Design review of the part built by this model. Coordinates are the model's own, in mm. A direction names the side the tool comes from. Coordinates: 2 decimals unless noted, no trailing zeros. Order: outer loops, then holes, each group sorted by start corner. A loop starts at its lowest first (then second) coordinate and runs counter-clockwise, first axis right, second up. Notation, with made-up numbers: (54, 60.25) - (100, 60.25) arc R19 ccw to (100, 85.25) - close; hole circle Ø8 at (-4, -30). An arc over 180 degrees is marked (long way). Write item = value, one per line. Start each with the question number.
```python
from build123d import *
from OCP.BRepFilletAPI import BRepFilletAPI_MakeChamfer

# Parameters (mm, degrees)
AUFSATZ_LINEAR_AUSTRAGEN1_DEPTH = 45
FASE1_SIZE                      = 35
FASE1_SIZE2                     = 50
FASE2_SIZE                      = 35
FASE2_SIZE2                     = 5
SCHNITT_LINEAR_AUSTRAGEN2_DEPTH = 140.810416962
SKIZZE4_W                       = 210
SKIZZE4_H                       = 7
AUFSATZ_LINEAR_AUSTRAGEN2_DEPTH = 10
VERRUNDUNG2_R                   = 3.5
VERRUNDUNG3_R                   = 3


with BuildPart() as part:
    # Skizze1 → Aufsatz-Linear austragen1 (new body)
    with BuildSketch(Plane(origin=(0, 0, 0), x_dir=(1, 0, 0), z_dir=(0, 1, 0))):
        Polygon((-105, -55), (-105, 0), (105, 0), (105, -55), (110, -55), (120.403291862, 4), (-120.403291862, 4), (-110, -55), align=None)
    extrude(amount=AUFSATZ_LINEAR_AUSTRAGEN1_DEPTH)

    # Fase1: one chamfer whose edges measure the first distance from different faces: ONE call of the kernel's chamfer builder (chamfer() names one face for all edges)
    fase1_edges_1 = [part.edges().sort_by_distance(p)[0] for p in [
        (107.5, 45, 55),
    ]]
    fase1_side_1 = [part.faces().sort_by_distance(p)[0] for p in [
        (107.5, 22.5, 55),
    ]]
    fase1_edges_2 = [part.edges().sort_by_distance(p)[0] for p in [
        (-107.5, 45, 55),
    ]]
    fase1_side_2 = [part.faces().sort_by_distance(p)[0] for p in [
        (-107.5, 22.5, 55),
    ]]
    fase1 = BRepFilletAPI_MakeChamfer(part.part.solid().wrapped)
    for e in fase1_edges_1:
        fase1.Add(FASE1_SIZE, FASE1_SIZE2, e.wrapped, fase1_side_1[0].wrapped)  # the first distance lies on this face
    for e in fase1_edges_2:
        fase1.Add(FASE1_SIZE, FASE1_SIZE2, e.wrapped, fase1_side_2[0].wrapped)  # the first distance lies on this face
    add(Compound.cast(fase1.Shape()), mode=Mode.REPLACE)

    # Fase2: one chamfer whose edges measure the first distance from different faces: ONE call of the kernel's chamfer builder (chamfer() names one face for all edges)
    fase2_edges_1 = [part.edges().sort_by_distance(p)[0] for p in [
        (-119.609820449, 45, 0.5),
    ]]
    fase2_side_1 = [part.faces().sort_by_distance(p)[0] for p in [
        (-116.314008321, 17.174625468, 19.191479401),
    ]]
    fase2_edges_2 = [part.edges().sort_by_distance(p)[0] for p in [
        (119.609820449, 45, 0.5),
    ]]
    fase2_side_2 = [part.faces().sort_by_distance(p)[0] for p in [
        (116.314008321, 17.174625468, 19.191479401),
    ]]
    fase2 = BRepFilletAPI_MakeChamfer(part.part.solid().wrapped)
    for e in fase2_edges_1:
        fase2.Add(FASE2_SIZE, FASE2_SIZE2, e.wrapped, fase2_side_1[0].wrapped)  # the first distance lies on this face
    for e in fase2_edges_2:
        fase2.Add(FASE2_SIZE, FASE2_SIZE2, e.wrapped, fase2_side_2[0].wrapped)  # the first distance lies on this face
    add(Compound.cast(fase2.Shape()), mode=Mode.REPLACE)

    # Skizze2 → Schnitt-Linear austragen2 (cut, through all)
    with BuildSketch(Plane.XY):
        Polygon((-105, 45), (-61.698729811, 20), (61.698729811, 20), (105, 45), align=None)
    extrude(amount=-SCHNITT_LINEAR_AUSTRAGEN2_DEPTH, mode=Mode.SUBTRACT)

    # Skizze4 → Aufsatz-Linear austragen2 (add)
    with BuildSketch(Plane(origin=(0, 0, 0), x_dir=(1, 0, 0), z_dir=(0, 1, 0))):
        with Locations((0, -48.5)):
            Rectangle(SKIZZE4_W, SKIZZE4_H)
        with Locations((0, -22.5)):
            Rectangle(SKIZZE4_W, SKIZZE4_H)
    extrude(amount=AUFSATZ_LINEAR_AUSTRAGEN2_DEPTH)

    # Verrundung2
    verrundung2_edges = [part.edges().sort_by_distance(p)[0] for p in [
        (0, 10, 52),
        (0, 10, 45),
        (0, 10, 19),
        (0, 10, 26),
    ]]
    fillet(verrundung2_edges, radius=VERRUNDUNG2_R - 0.0001)  # a hair under: the kernel refuses the full size

    # Verrundung3
    verrundung3_edges = [part.edges().sort_by_distance(p)[0] for p in [
        (-105, 8.974903023, 24.974903023),
        (105, 3.25005, 52),
        (-105, 3.25005, 52),
        (-105, 3.25005, 45),
        (105, 3.25005, 45),
        (-105, 3.25005, 19),
        (105, 3.25005, 19),
        (105, 3.25005, 26),
        (-105, 3.25005, 26),
        (105, 8.974903023, 50.974903023),
        (-105, 8.974903023, 50.974903023),
        (-105, 8.974903023, 46.025096977),
        (105, 8.974903023, 46.025096977),
        (-105, 8.974903023, 20.025096977),
        (105, 8.974903023, 20.025096977),
        (105, 8.974903023, 24.974903023),
    ]]
    fillet(verrundung3_edges, radius=VERRUNDUNG3_R - 0.0001)  # a hair under: the kernel refuses the full size


solid = part.part
```
Item 1: For line 1 (X direction, y = 38, z = 1.5); line 2 (Z direction, x = -60.5, y = 7.5); line 3 (Y direction, x = -20, z = -1), list the stretches that pass through material, from the lowest coordinate up.
Item 2: Add section C-C on y = 35.5. Give the boundary of the cut face in (x, z).
Item 3: For P1, Ø12, axis at y = 13, z = 19.5, coming from the -X side; P2, Ø3.5, axis at x = 30.5, y = 4.5, coming from the +Z side; P3, Ø22.5, axis at y = 11.5, z = 27, coming from the +X side, all flat-tipped, find the tip position at first contact; note any pin that passes through.
Item 4: For faces 1 (the flat face through (-1, 20, -2)), 2 (the flat face through (-1, 12, 0)), 3 (the flat face through (-105, 17, 16)), list the 3-axis set-ups (+Z, -Z, +X, -X, +Y, -Y) from which the entire face can be reached by the end or side of a thin tool; tool diameter is ignored.
Item 5: Add section A-A on x = 40.5. State how many separate pieces and enclosed holes the cut face has, plus the area to 3 significant figures.
Item 6: Add section B-B on z = 7.5. Give the boundary of the cut face in (x, y), plus the area to 3 significant figures.
Item 7: Mouldability with a two-part tool opening along X and no side actions: class faces 4 (the flat face through (108.337, 27.745, 29.65)), 5 (the flat face through (114.335, 23.856, 19.014)), 6 (the flat face through (-1, 3, 52)), 7 (the flat face through (-83.652, 32.675, -1.972)) as +X half, -X half, draft (parallel to the pull), parting line (faces both ways), or undercut.
Worked out:
q1.line_1 = -115.37 to -105, 105 to 115.37
q1.line_2 = -4 to 0, 19.15 to 25.85, 45.15 to 51.85
q1.line_3 = 0 to 20
q2.outline = (-116.7, -4) - (-88.55, -4) - (-88.55, 0) - (-105, 0) - (-105, 18.57) - (-112.72, 18.57) - close; (88.55, -4) - (116.7, -4) - (112.72, 18.57) - (105, 18.57) - (105, 0) - (88.55, 0) - close
q3.P1 = -117.18
q3.P2 = 52
q3.P3 = 116.9
q4.face_1 = +Z, -Z, +Y
q4.face_2 = +Y, -Y
q4.face_3 = +Y
q5.separate_pieces = 3
q5.enclosed_holes = 0
q5.area = 209 mm2
q6.outline = (-118.38, 0) - (-105, 0) - (-105, 43.25) - (-113.55, 43.25) - (-118.38, 10) - close; (105, 0) - (118.38, 0) - (118.38, 10) - (113.55, 43.25) - (105, 43.25) - close
q6.area = 997 mm2
q7.face_4 = draft
q7.face_5 = +X half
q7.face_6 = undercut
q7.face_7 = undercut
